Geometry: final body of the model. Coordinates: model frame, mm. Face numbers are marked on the shaded views. Give positions to 0.01 mm unless a question says otherwise; leave off trailing zeros. Loops run counter-clockwise (first coordinate to the right, second up) from the corner with the lowest first, then second, coordinate; pieces in that order, holes last. Notation, with made-up numbers: (70.25, 55.25) -> (98.25, 55.25) arc R17 ccw to (98.25, 78.25) -> close; hole circle Ø10 at (78, 18). An arc over 180 degrees is marked (long way). One line per question, with ' | ' between items. Start each with the question number.
Item 1: Section A-A on x = 0. Return loops of the section in (y, z).
Item 2: Section B-B on x = -53. Return loops of the section in (y, z).
Item 3: Material intervals for line 1 along Y through (x, z) = (0, 16); line 2 along Y through (x, z) = (0, 9); line 3 along Z through (x, y) = (-37.5, 38.5), sorted ascending. Write a range as [from, to].
Item 4: Section C-C on z = -17.5. Return loops of the section in (x, y), then the cut area to 3 significant figures.
Item 5: Mould query, pull axis Y, two halves, no side actions, for the marked faces 1, 2 and 3. Classes: released by +Y, released by -Y, zero draft, split by the parting line, or undercut.
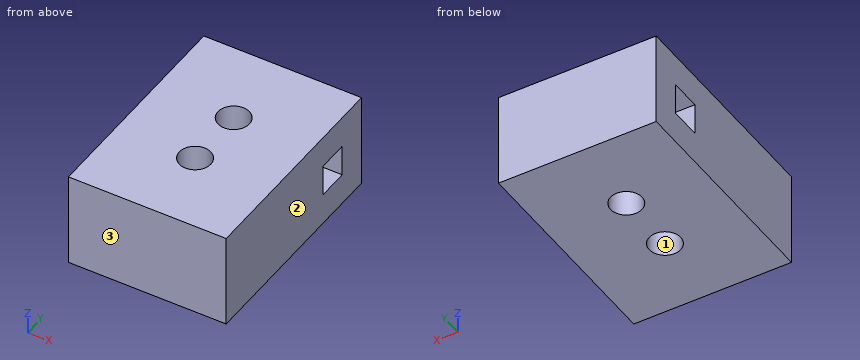
from build123d import *

# Parameters (mm, degrees)
F0_W     = 127
F0_H     = 177.8
F1_DEPTH = 38.1
F2_R     = 12.7
F3_DEPTH = 76.201
F4_W     = 25.4
F4_H     = 25.4
F5_DEPTH = 127.001


with BuildPart() as f1:
    # F0 (on Top) → F1 (new body, symmetric)
    with BuildSketch(Plane.XY):
        Rectangle(F0_W, F0_H)
    extrude(amount=F1_DEPTH, both=True)

    # F2 (on face) → F3 (cut, through all)
    with BuildSketch(Plane.XY.offset(38.1)):
        with Locations((0, 24.567431)):
            Circle(F2_R)
        with Locations((0, -26.232569)):
            Circle(F2_R)
    extrude(amount=-F3_DEPTH, mode=Mode.SUBTRACT)

    # F4 (on face) → F5 (cut, through all)
    with BuildSketch(Plane.YZ.offset(63.5)):
        with Locations((50.8, 0)):
            Rectangle(F4_W, F4_H)
    extrude(amount=-F5_DEPTH, mode=Mode.SUBTRACT)


solid = f1.part
Result sheet:
1) outline: (-88.9, -38.1) -> (-38.93, -38.1) -> (-38.93, 38.1) -> (-88.9, 38.1) -> close; (-13.53, -38.1) -> (11.87, -38.1) -> (11.87, 38.1) -> (-13.53, 38.1) -> close; (37.27, -38.1) -> (88.9, -38.1) -> (88.9, 38.1) -> (37.27, 38.1) -> close; hole (38.1, -12.7) -> (63.5, -12.7) -> (63.5, 12.7) -> (38.1, 12.7) -> close
2) outline: (-88.9, -38.1) -> (88.9, -38.1) -> (88.9, 38.1) -> (-88.9, 38.1) -> close; hole (38.1, -12.7) -> (63.5, -12.7) -> (63.5, 12.7) -> (38.1, 12.7) -> close
3) line 1: y = [-88.9, -38.93], [-13.53, 11.87], [37.27, 88.9] | line 2: y = [-88.9, -38.93], [-13.53, 11.87], [37.27, 38.1], [63.5, 88.9] | line 3: z = [-38.1, -12.7], [12.7, 38.1]
4) outline: (-63.5, -88.9) -> (63.5, -88.9) -> (63.5, 88.9) -> (-63.5, 88.9) -> close; hole circle Ø25.4 at (0, -26.23); hole circle Ø25.4 at (0, 24.57) | area: 21,600 mm²
5) face 1: undercut | face 2: zero draft | face 3: released by -Y
